Design review of the part shown in the three views and the two pictorial views. Dimensions are in mm from the part's minimum x, y and z. A direction names the side the tool comes from. Give positions to 0.01 mm unless a question says otherwise; leave off trailing zeros. Order: outer loops, then holes, each group sorted by start corner. A loop starts at its lowest first (then second) coordinate and runs counter-clockwise, first axis right, second up. Notation, with made-up numbers: (34.5, 81.25) -> (38.5, 81.25) arc R14 cw to (38.5, 108.25) -> close; hole circle Ø7 at (-6.75, -27). An arc over 180 degrees is marked (long way). Answer in a Markdown table with one row per item. Add a question column.
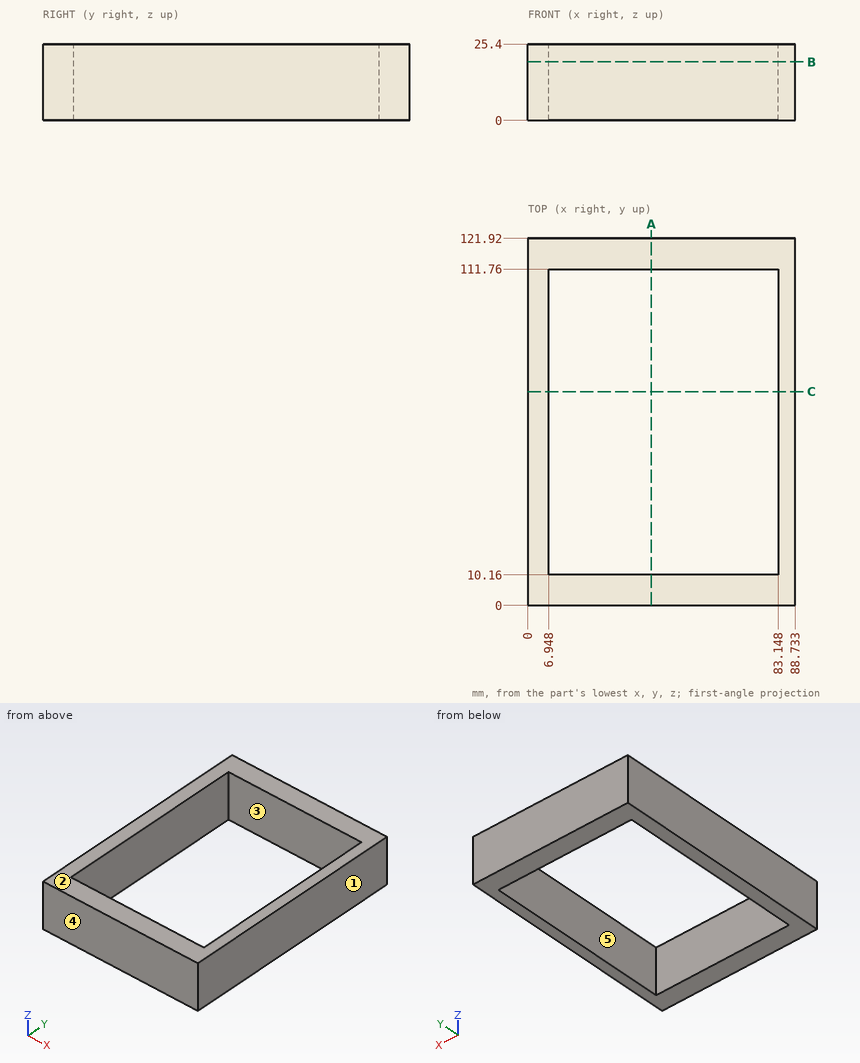
1) Add section C-C, the plane y = 71. Write out the cut boundary in (x, z).
2) Clearance check with a flat-ended pin moving along its axis: P1, Ø7.5, axis at y = 47, z = 11, coming from the -X side. State where the tip first meets the part, or that it passes through.
3) Add section A-A, the plane x = 41. Write out the cut boundary in (y, z).
4) Mouldability with a two-part tool opening along X and no side actions: class the marked faces 1, 2 and 3 as +X half, -X half, draft (parallel to the pull), parting line (faces both ways), or undercut.
5) For L1, parallel to Y at x = 47, z = 9.5; L2, parallel to X at y = 92, z = 6.5, list the stretches that pass through material, from the lowest coordinate up.
6) Machinability: for the marked faces 4 and 5, which of the approach directions +Z, -Z, +X, -X, +Y, -Y give a long, thin tool a straight path to every point of the face, cutting with its end or side? Answer none if there is none.
7) Add section B-B, the plane z = 19.5. Write out the cut boundary in (x, y).
Verdict:
| question | item | result |
|---|---|---|
| 1 | outline | (0, 0) -> (6.95, 0) -> (6.95, 25.4) -> (0, 25.4) -> close; (83.15, 0) -> (88.73, 0) -> (88.73, 25.4) -> (83.15, 25.4) -> close |
| 2 | P1 | stops at x = 0 |
| 3 | outline | (0, 0) -> (10.16, 0) -> (10.16, 25.4) -> (0, 25.4) -> close; (111.76, 0) -> (121.92, 0) -> (121.92, 25.4) -> (111.76, 25.4) -> close |
| 4 | face 1 | +X half |
| 4 | face 2 | draft |
| 4 | face 3 | undercut |
| 5 | L1 | y = 0 to 10.16, 111.76 to 121.92 |
| 5 | L2 | x = 0 to 6.95, 83.15 to 88.73 |
| 6 | face 4 | +Z, -Z, +X, -X, -Y |
| 6 | face 5 | +Z, -Z |
| 7 | outline | (0, 0) -> (88.73, 0) -> (88.73, 121.92) -> (0, 121.92) -> close; hole (6.95, 10.16) -> (83.15, 10.16) -> (83.15, 111.76) -> (6.95, 111.76) -> close |
